CAD build for the part. Positions are in the model's coordinates, mm. A direction names the side the tool comes from. Give positions to 0.01 mm unless a question says otherwise; leave off trailing zeros. Write each loop counter-clockwise with the first axis right and the second up, starting at its lowest first coordinate (ties: lowest second). Pieces come first, ordered by that corner, then holes. Notation, with made-up numbers: (-33, 89.5) -> (4, 89.5) arc R25 ccw to (4, 113.5) -> close; hole circle Ø1 at (-1.5, 28.5). An arc over 180 degrees is marked (long way). Answer as a JSON object with one key per item and string values.
```python
from build123d import *

# Parameters (mm, degrees)
EXTRUDE_1_DEPTH = 290
SKETCH_2_W      = 598
SKETCH_2_H      = 2
EXTRUDE_2_DEPTH = 800
EXTRUDE_START   = 801.875465
SKETCH_3_W      = 600
SKETCH_3_H      = 2
EXTRUDE_3_DEPTH = 550


with BuildPart() as part:
    # 草图1 → 凸台-拉伸1 (new body)
    with BuildSketch(Plane.XY):
        Polygon((0, 801.875465042), (1.875465042, 801.875465042), (391.533669143, 801.875465042), (391.533669143, 803.750930084), (504.06157166, 803.750930084), (504.06157166, 801.875465042), (451.987075109, 801.875465042), (451.987075109, 800), (1.875465042, 800), (1.875465042, 2), (598, 2), (598, 802), (600, 802), (600, 1.871806921), (600, 0), (0, 0), (0, 1.875465042), align=None)
    extrude(amount=EXTRUDE_1_DEPTH)

    # 草图2 → 凸台-拉伸2 (add)
    with BuildSketch(Plane(origin=(0, 0, 0), x_dir=(1, 0, 0), z_dir=(0, 1, 0))):
        with Locations((299, -1)):
            Rectangle(SKETCH_2_W, SKETCH_2_H)
    extrude(amount=EXTRUDE_2_DEPTH)

    # 草图3 → 凸台-拉伸3 (add)
    with BuildSketch(Plane(origin=(0, 0, 0), x_dir=(1, 0, 0), z_dir=(0, 1, 0)).offset(EXTRUDE_START)):
        with Locations((300, -289)):
            Rectangle(SKETCH_3_W, SKETCH_3_H)
    extrude(amount=-EXTRUDE_3_DEPTH)


solid = part.part
```
1) Slice it at D-D (y = 464.5). List the corners of the cut face in (x, z), then the cut area to 3 significant figures.
Model answer:
{"outline": "(0, 0) -> (600, 0) -> (600, 290) -> (0, 290) -> close; hole (1.88, 2) -> (598, 2) -> (598, 288) -> (1.88, 288) -> close", "area": "3,510 mm2"}
2) 3-axis set-ups, long thin cutter, end or side, ignore diameter. For faces 1 (the flat face through (296, 2, 144)), 2 (the flat face through (478, 801.875, 142)), 3 (the flat face through (230, 800, 143)): which of +Z, -Z, +X, -X, +Y, -Y reach the whole face in a straight line?
Model answer:
{"face 1": "+Z", "face 2": "-Z", "face 3": "none"}
3) Mould opens along Z. For faces 4 (the flat face through (447, 803.751, 143)), 5 (the flat face through (296, 395, 2)), 6 (the flat face through (304, 497, 290)) say: released by +Z, released by -Z, zero draft, split by the parting line, or undercut.
Model answer:
{"face 4": "zero draft", "face 5": "undercut", "face 6": "released by +Z"}
4) Slice it at A-A (x = 473). List the corners of the cut face in (y, z), then the cut area to 3 significant figures.
Model answer:
{"outline": "(0, 0) -> (800, 0) -> (800, 2) -> (2, 2) -> (2, 290) -> (0, 290) -> close; (251.88, 288) -> (801.88, 288) -> (801.88, 0) -> (803.75, 0) -> (803.75, 290) -> (251.88, 290) -> close", "area": "3,820 mm2"}
5) Pin check, flat tips, straight feed: pin 1 (1 mm diameter, centred on x = 517, z = 163, fed in from +Y); pin 2 (1.5 mm diameter, centred on y = 803, z = 195, fed in from -X); pin 3 (1.6 mm diameter, centred on x = 532, z = 0.5, fed in from +Y). Stop position of each tip, or through.
Model answer:
{"pin 1": "stops at y = 2", "pin 2": "stops at x = 391.53", "pin 3": "stops at y = 800"}
6) Slice it at C-C (y = 116). List the corners of the cut face in (x, z).
Model answer:
{"outline": "(0, 0) -> (600, 0) -> (600, 290) -> (598, 290) -> (598, 2) -> (1.88, 2) -> (1.88, 290) -> (0, 290) -> close"}
7) Wall check: probe 1 along Y at (x, z) = (294.5, 25); probe 2 along Y at (x, z) = (480, 237); probe 3 along X at (y, z) = (769, 242.5). Give the ranges that are in metal, low to high.
Model answer:
{"probe 1": "y = 0 to 2, 800 to 801.88", "probe 2": "y = 0 to 2, 801.88 to 803.75", "probe 3": "x = 0 to 1.88, 598 to 600"}
8) Slice it at B-B (z = 121.5). List the corners of the cut face in (x, y), then the cut area to 3 significant figures.
Model answer:
{"outline": "(0, 0) -> (600, 0) -> (600, 802) -> (598, 802) -> (598, 2) -> (1.88, 2) -> (1.88, 800) -> (451.99, 800) -> (451.99, 801.88) -> (504.06, 801.88) -> (504.06, 803.75) -> (391.53, 803.75) -> (391.53, 801.88) -> (0, 801.88) -> close", "area": "5,360 mm2"}
